Source: CAD feature listing. Evaluate the final solid. Frame: model axes, mm. A direction names the side the tool comes from. Round coordinates to 2 decimals unless told otherwise and drop trailing zeros. Write each loop counter-clockwise with the first axis right and the second up, starting at its lowest first coordinate (ties: lowest second). Pieces come first, ordered by that corner, then holes. Notation, with made-up numbers: (-5, 67) -> (11, 67) arc R23 ccw to (11, 81) -> close; hole circle Ø3 at (35, -36.75). An arc over 180 degrees is marked (long way). Return JSON: item names as keys, results as strings. Group by question number.
from build123d import *

# Parameters (mm, degrees)
F4_R      = 3.683
F5_DEPTH  = 334.01
F6_R      = 3.683
F7_DEPTH  = 25.4
F8_R      = 6.35
F9_DEPTH  = 9.4742
F11_DEPTH = 24.765
F12_R     = 6.35
F13_DEPTH = 12.446


# Not quite as in the source:
# - a feature names something its author has since deleted; it is built from what else it names


with BuildPart() as f2:
    # F2: sweep along a path in F0
    with BuildLine(Plane.XZ) as f2_path:
        Line((0, 0), (0, 104.902))
        ThreePointArc((0, 104.902), (0.1125182852, 108.5847531474), (0.4496534022, 112.2537681409))
        Line((0.4496534022, 112.2537681409), (46.8818732396, 490.4138519163))
        ThreePointArc((46.8818732396, 490.4138519163), (69.6174413383, 530.5988324867), (114.1089879783, 542.9374303731))
        Line((114.1089879783, 542.9374303731), (117.890588816, 542.4731081747))
    # F1 (on Top) → F2 (sweep)
    with BuildSketch(Plane.XY):
        with BuildLine():
            ThreePointArc((-9.525, -6.35), (-8.5950640303, -8.5950640303), (-6.35, -9.525))
            Line((-6.35, -9.525), (6.35, -9.525))
            ThreePointArc((6.35, -9.525), (8.5950640303, -8.5950640303), (9.525, -6.35))
            Line((9.525, -6.35), (9.525, 6.35))
            ThreePointArc((9.525, 6.35), (8.5950640303, 8.5950640303), (6.35, 9.525))
            Line((6.35, 9.525), (-6.35, 9.525))
            ThreePointArc((-6.35, 9.525), (-8.5950640303, 8.5950640303), (-9.525, 6.35))
            Line((-9.525, 6.35), (-9.525, -6.35))
        make_face()
        with BuildLine():
            Line((5.461, -6.477), (-5.461, -6.477))
            ThreePointArc((-5.461, -6.477), (-6.1794204897, -6.1794204897), (-6.477, -5.461))
            Line((-6.477, -5.461), (-6.477, 5.461))
            ThreePointArc((-6.477, 5.461), (-6.1794204897, 6.1794204897), (-5.461, 6.477))
            Line((-5.461, 6.477), (5.461, 6.477))
            ThreePointArc((5.461, 6.477), (6.1794204897, 6.1794204897), (6.477, 5.461))
            Line((6.477, 5.461), (6.477, -5.461))
            ThreePointArc((6.477, -5.461), (6.1794204897, -6.1794204897), (5.461, -6.477))
        make_face(mode=Mode.SUBTRACT)
    sweep(path=f2_path.line)

    # F4 (on Front) → F5 (cut, symmetric)
    with BuildSketch(Plane.XZ):
        with Locations((0, 22.225)):
            Circle(F4_R)
    extrude(amount=F5_DEPTH, both=True, mode=Mode.SUBTRACT)

    # F6 (on face) → F7 (cut)
    with BuildSketch(Plane(origin=(-22.5893491944, 0, 2.7736233219), x_dir=(0, -1, 0), z_dir=(-0.9925461516, 0, 0.1218693434))):
        with Locations((0, 464.5318445404)):
            Circle(F6_R)
    extrude(amount=-F7_DEPTH, mode=Mode.SUBTRACT)

    # F8 (on face) → F9 (cut)
    with BuildSketch(Plane(origin=(-22.5893491944, 0, 2.7736233219), x_dir=(0, -1, 0), z_dir=(-0.9925461516, 0, 0.1218693434))):
        with Locations((0, 464.5318445404)):
            Circle(F8_R)
    extrude(amount=-F9_DEPTH, mode=Mode.SUBTRACT)

    # F10 (on face) → F11 (join)
    with BuildSketch(Plane(origin=(50.5216003355, 0, -6.2032725133), x_dir=(0, 1, 0), z_dir=(0.9925461516, 0, -0.1218693434))):
        with BuildLine():
            ThreePointArc((9.525, 559.1468445404), (8.5950640303, 561.3919085707), (6.35, 562.3218445404))
            Line((6.35, 562.3218445404), (-6.35, 562.3218445404))
            ThreePointArc((-6.35, 562.3218445404), (-8.5950640303, 561.3919085707), (-9.525, 559.1468445404))
            Line((-9.525, 559.1468445404), (-9.525, 546.4468445404))
            ThreePointArc((-9.525, 546.4468445404), (-8.5950640303, 544.2017805101), (-6.35, 543.2718445404))
            Line((-6.35, 543.2718445404), (6.35, 543.2718445404))
            ThreePointArc((6.35, 543.2718445404), (8.5950640303, 544.2017805101), (9.525, 546.4468445404))
            Line((9.525, 546.4468445404), (9.525, 559.1468445404))
        make_face()
        with BuildLine():
            ThreePointArc((-6.477, 558.2578445404), (-6.1794204897, 558.9762650301), (-5.461, 559.2738445404))
            Line((-5.461, 559.2738445404), (5.461, 559.2738445404))
            ThreePointArc((5.461, 559.2738445404), (6.1794204897, 558.9762650301), (6.477, 558.2578445404))
            Line((6.477, 558.2578445404), (6.477, 547.3358445404))
            ThreePointArc((6.477, 547.3358445404), (6.1794204897, 546.6174240507), (5.461, 546.3198445404))
            Line((5.461, 546.3198445404), (-5.461, 546.3198445404))
            ThreePointArc((-5.461, 546.3198445404), (-6.1794204897, 546.6174240507), (-6.477, 547.3358445404))
            Line((-6.477, 547.3358445404), (-6.477, 558.2578445404))
        make_face(mode=Mode.SUBTRACT)
    extrude(amount=F11_DEPTH)

    # F12 (on face) → F13 (cut)
    with BuildSketch(Plane(origin=(0, 9.525, 0), x_dir=(-1, 0, 0), z_dir=(0, 1, 0))):
        with Locations((0, 22.225)):
            Circle(F12_R)
    extrude(amount=-F13_DEPTH, mode=Mode.SUBTRACT)


solid = f2.part
Item 1: Set-up query: faces 4 (the flat face through (33, 9.525, 327)), 5 (the cylindrical face through (17.85, -6.17, 304.73)), 6 (the flat face through (9.525, 0, 53)), 7 (the cylindrical face through (6.344, 7.763, 22.504)), 8 (the flat face through (12.81, 0.09, 291.08)). Return all of +Z, -Z, +X, -X, +Y, -Y with unobstructed straight access to the full face (end or side cutting, diameter ignored); none if empty.
Item 2: Cut plane B-B on y = -0.75. Give the number of separate pieces and of enclosed holes in the cut face, and give its area (3 significant figures).
Item 3: Cut plane A-A on z = 53.5. Output: boundary loops of the cut face in (x, y) (3 decimals), and give its area (3 significant figures).
Item 4: Pull-direction query (Z, two-part tool) for faces 1 (the flat face through (33.445, -0.089, 302.82)), 2 (the flat face through (36.128, 0.089, 480.984)), 3 (the flat face through (30, 6.477, 331)); classes: +Z half, -Z half, draft (parallel to the pull), parting line (faces both ways), or undercut.
Item 5: Material intervals for probe 1 along Y at (x, z) = (14.5, 188.5) (3 decimals); probe 2 along X at (y, z) = (-6.75, 237.5), sorted ascending.
Item 6: First-contact query: pin 1 Ø8.5 at (y, z) = (-2.5, 58) entering from +X (3 decimals); pin 2 Ø8 at (y, z) = (2.5, 460) entering from +X; pin 3 Ø6 at (y, z) = (2.5, 356) entering from +X. Flat tips, straight axial feed; report the tip coordinate or a pass-through.
Here are the results:
{
 "1": {"face 4": "+Z, -Z, +X, -X, +Y", "face 5": "none", "face 6": "-Z, +X, +Y, -Y", "face 7": "+Y", "face 8": "+Z, -X, +Y, -Y"},
 "2": {"separate pieces": "4", "enclosed holes": "0", "area": "3,700 mm^2"},
 "3": {"outline": "(-9.525, -6.35) arc R3.175 ccw to (-6.35, -9.525) -> (6.35, -9.525) arc R3.175 ccw to (9.525, -6.35) -> (9.525, 6.35) arc R3.175 ccw to (6.35, 9.525) -> (-6.35, 9.525) arc R3.175 ccw to (-9.525, 6.35) -> close; hole (-6.477, -5.461) arc R1.016 ccw to (-5.461, -6.477) -> (5.461, -6.477) arc R1.016 ccw to (6.477, -5.461) -> (6.477, 5.461) arc R1.016 ccw to (5.461, 6.477) -> (-5.461, 6.477) arc R1.016 ccw to (-6.477, 5.461) -> close", "area": "187 mm^2"},
 "4": {"face 1": "-Z half", "face 2": "+Z half", "face 3": "undercut"},
 "5": {"probe 1": "y = -9.525 to -6.477, 6.477 to 9.525", "probe 2": "x = 6.26 to 25.4"},
 "6": {"pin 1": "stops at x = 9.525", "pin 2": "stops at x = 53.23", "pin 3": "stops at x = 40.34"}
}
